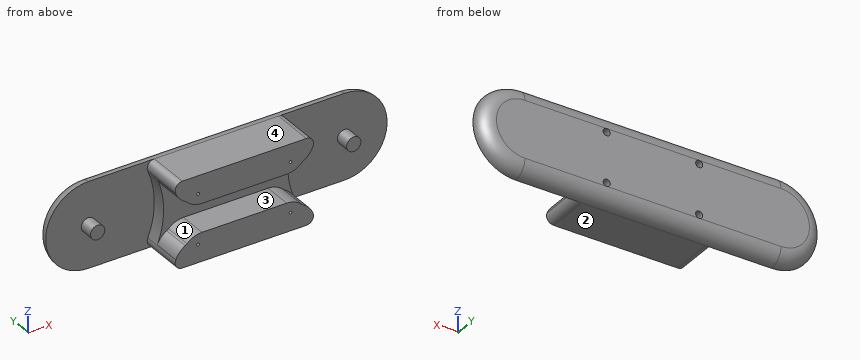
from build123d import *

# Parameters (mm, degrees)
BOSS_EXTRUDE1_DEPTH     = 40
FILLET1_R               = 10
CUT_EXTRUDE1_DEPTH      = 30
SKETCH4_R               = 5
BOSS_EXTRUDE3_DEPTH     = 10
CUT_EXTRUDE2_REACH      = 181.038
CUT_EXTRUDE2_END_RADIUS = 60
SKETCH5_W               = 20
SKETCH5_H               = 40
FILLET2_R               = 5
CUT_EXTRUDE3_REACH      = 153.142
SKETCH6_R               = 1
SKETCH7_R               = 2.5
CUT_EXTRUDE4_DEPTH      = 5
SKETCH8_R               = 6
CUT_EXTRUDE5_DEPTH      = 20
FILLET3_R               = 15


with BuildPart() as part:
    # Sketch1 → Boss-Extrude1 (new body)
    with BuildSketch(Plane(origin=(0, 0, 0), x_dir=(1, 0, 0), z_dir=(0, 1, 0))):
        with BuildLine():
            Line((-67.694698117, 31.515169882), (112.305301883, 31.515169882))
            ThreePointArc((112.305301883, 31.515169882), (142.305301883, 1.515169882), (112.305301883, -28.484830118))
            Line((112.305301883, -28.484830118), (-67.694698117, -28.484830118))
            ThreePointArc((-67.694698117, -28.484830118), (-97.694698117, 1.515169882), (-67.694698117, 31.515169882))
        make_face()
    extrude(amount=BOSS_EXTRUDE1_DEPTH)

    # Fillet1
    fillet1_edges = [part.edges().sort_by_distance(p)[0] for p in [
        (142.305301883, 40, -1.515169882),
        (22.305301883, 40, -31.515169882),
        (-97.694698117, 40, -1.515169882),
        (22.305301883, 40, 28.484830118),
    ]]
    fillet(fillet1_edges, radius=FILLET1_R)

    # Sketch3 → Cut-Extrude1 (cut)
    with BuildSketch(Plane.XZ):
        with BuildLine():
            Line((73.949041486, -31.515169882), (148.949041486, -31.515169882))
            Line((148.949041486, -31.515169882), (148.949041486, 28.484830118))
            Line((148.949041486, 28.484830118), (73.949041486, 28.484830118))
            ThreePointArc((73.949041486, 28.484830118), (65.910565713, -1.515169882), (73.949041486, -31.515169882))
        make_face()
        with BuildLine():
            Line((-29.33843772, 28.484830118), (-104.33843772, 28.484830118))
            Line((-104.33843772, 28.484830118), (-104.33843772, -31.515169882))
            Line((-104.33843772, -31.515169882), (-29.33843772, -31.515169882))
            ThreePointArc((-29.33843772, -31.515169882), (-21.299961947, -1.515169882), (-29.33843772, 28.484830118))
        make_face()
    extrude(amount=-CUT_EXTRUDE1_DEPTH, mode=Mode.SUBTRACT)

    # Sketch4 → Boss-Extrude3 (add)
    with BuildSketch(Plane(origin=(0, 30, 0), x_dir=(-1, 0, 0), z_dir=(0, -1, 0))):
        with Locations(Location((-112.305301883, 1.515169882, 0), (0, 0, 90))):
            Circle(SKETCH4_R)
        with Locations(Location((67.694698117, 1.515169882, 0), (0, 0, 270))):
            Circle(SKETCH4_R)
    extrude(amount=BOSS_EXTRUDE3_DEPTH)

    # Cut-Extrude2: up to this cylinder (the profile starts outside it)
    cut_extrude2_end = Plane(origin=(-81.299961947, 0, -1.515169882), z_dir=(0, -1, 0)) * Cylinder(CUT_EXTRUDE2_END_RADIUS, 483.076, mode=Mode.PRIVATE)
    # Sketch5 → Cut-Extrude2 (cut, up to the surface)
    with BuildSketch(Plane(origin=(73.949041486, 0, 0), x_dir=(0, 0, -1), z_dir=(1, 0, 0)), mode=Mode.PRIVATE) as cut_extrude2_sk1:
        with Locations((1.515169882, 0)):
            Rectangle(SKETCH5_W, SKETCH5_H)
    cut_extrude2_tool1 = extrude(cut_extrude2_sk1.sketch, amount=-CUT_EXTRUDE2_REACH, mode=Mode.PRIVATE) - cut_extrude2_end
    add(cut_extrude2_tool1.solids().sort_by_distance((73.949041, 0, -1.51517))[0], mode=Mode.SUBTRACT)

    # Fillet2
    # the kernel refuses this fillet: 5 mm, written as the material it takes off along each edge
    with BuildSketch(Plane(origin=(-29.33843772, -20.096189432, 28.484830118), x_dir=(0.44322659401027775, 0, -0.8964096085841831), z_dir=(0, 1, 0))) as fillet2_piece_1:
        with BuildLine():
            CenterArc((8.044914281, -4.989633951), FILLET2_R, 93.690067526, 112.619864948)
            Line((3.562866238, -7.205766921), (0, 0))
            ThreePointArc((0, 0), (3.861558855, -0.124392586), (7.72311771, 0))
        make_face()
    extrude(amount=50.096189432, mode=Mode.SUBTRACT)
    with BuildSketch(Plane(origin=(-29.33843772, -20.096189432, -31.515169882), x_dir=(1, 0, 0), z_dir=(0, 1, 0))) as fillet2_piece_2:
        with BuildLine():
            CenterArc((8.038475773, -5), FILLET2_R, 90, 112.619864948)
            ThreePointArc((3.423091158, -6.923076923), (1.823052288, -3.406404359), (0, 0))
            Line((0, 0), (8.038475773, 0))
        make_face()
    extrude(amount=50.096189432, mode=Mode.SUBTRACT)
    with BuildSketch(Plane(origin=(73.949041486, -20.096189432, -31.515169882), x_dir=(-1, 0, 0), z_dir=(0, 1, 0))) as fillet2_piece_3:
        with BuildLine():
            CenterArc((8.038475773, 5), FILLET2_R, 157.380135052, 112.619864948)
            ThreePointArc((3.423091158, 6.923076923), (1.823052288, 3.406404359), (0, 0))
            Line((0, 0), (8.038475773, 0))
        make_face()
    extrude(amount=50.096189432, mode=Mode.SUBTRACT)
    with BuildSketch(Plane(origin=(73.949041486, -20.096189432, 28.484830118), x_dir=(-0.4432265940102763, 0, -0.8964096085841838), z_dir=(0, 1, 0))) as fillet2_piece_4:
        with BuildLine():
            CenterArc((8.044914281, 4.989633951), FILLET2_R, 153.690067526, 112.619864948)
            Line((3.562866238, 7.205766921), (0, 0))
            ThreePointArc((0, 0), (3.861558855, 0.124392586), (7.72311771, 0))
        make_face()
    extrude(amount=50.096189432, mode=Mode.SUBTRACT)

    # Sketch6 → Cut-Extrude3 (cut, up to next)
    with BuildSketch(Plane(origin=(0, 0, 0), x_dir=(-1, 0, 0), z_dir=(0, -1, 0)), mode=Mode.PRIVATE) as cut_extrude3_sk1:
        with Locations(Location((10.194698117, -15.984830118, 0), (0, 0, 90))):
            Circle(SKETCH6_R)
    cut_extrude3_tool1 = extrude(cut_extrude3_sk1.sketch, amount=-CUT_EXTRUDE3_REACH, mode=Mode.PRIVATE) & part.part
    # Sketch6 → Cut-Extrude3 (cut, up to next)
    with BuildSketch(Plane(origin=(0, 0, 0), x_dir=(-1, 0, 0), z_dir=(0, -1, 0)), mode=Mode.PRIVATE) as cut_extrude3_sk2:
        with Locations(Location((-54.805301883, -15.984830118, 0), (0, 0, 90))):
            Circle(SKETCH6_R)
    cut_extrude3_tool2 = extrude(cut_extrude3_sk2.sketch, amount=-CUT_EXTRUDE3_REACH, mode=Mode.PRIVATE) & part.part
    # Sketch6 → Cut-Extrude3 (cut, up to next)
    with BuildSketch(Plane(origin=(0, 0, 0), x_dir=(-1, 0, 0), z_dir=(0, -1, 0)), mode=Mode.PRIVATE) as cut_extrude3_sk3:
        with Locations(Location((-54.805301883, 19.015169882, 0), (0, 0, 90))):
            Circle(SKETCH6_R)
    cut_extrude3_tool3 = extrude(cut_extrude3_sk3.sketch, amount=-CUT_EXTRUDE3_REACH, mode=Mode.PRIVATE) & part.part
    # Sketch6 → Cut-Extrude3 (cut, up to next)
    with BuildSketch(Plane(origin=(0, 0, 0), x_dir=(-1, 0, 0), z_dir=(0, -1, 0)), mode=Mode.PRIVATE) as cut_extrude3_sk4:
        with Locations(Location((10.194698117, 19.015169882, 0), (0, 0, 90))):
            Circle(SKETCH6_R)
    cut_extrude3_tool4 = extrude(cut_extrude3_sk4.sketch, amount=-CUT_EXTRUDE3_REACH, mode=Mode.PRIVATE) & part.part
    add(cut_extrude3_tool1.solids().sort_by_distance((-10.194698, 0, 15.98483))[0], mode=Mode.SUBTRACT)
    add(cut_extrude3_tool2.solids().sort_by_distance((54.805302, 0, 15.98483))[0], mode=Mode.SUBTRACT)
    add(cut_extrude3_tool3.solids().sort_by_distance((54.805302, 0, -19.01517))[0], mode=Mode.SUBTRACT)
    add(cut_extrude3_tool4.solids().sort_by_distance((-10.194698, 0, -19.01517))[0], mode=Mode.SUBTRACT)

    # Sketch7 → Cut-Extrude4 (cut)
    with BuildSketch(Plane(origin=(0, 40, 0), x_dir=(1, 0, 0), z_dir=(0, 1, 0))):
        with Locations(Location((-10.194698117, 19.015169882, 0), (0, 0, 270))):
            Circle(SKETCH7_R)
        with Locations(Location((-10.194698117, -15.984830118, 0), (0, 0, 270))):
            Circle(SKETCH7_R)
        with Locations(Location((54.805301883, -15.984830118, 0), (0, 0, 270))):
            Circle(SKETCH7_R)
        with Locations(Location((54.805301883, 19.015169882, 0), (0, 0, 270))):
            Circle(SKETCH7_R)
    extrude(amount=-CUT_EXTRUDE4_DEPTH, mode=Mode.SUBTRACT)

    # Sketch8 → Cut-Extrude5 (cut)
    with BuildSketch(Plane.XZ):
        with Locations((-22.139164116, 8.484830118)):
            Circle(SKETCH8_R)
        with Locations((-22.139164116, -11.515169882)):
            Circle(SKETCH8_R)
        with Locations((66.749767882, -11.515169882)):
            Circle(SKETCH8_R)
        with Locations((66.749767882, 8.484830118)):
            Circle(SKETCH8_R)
    extrude(amount=-CUT_EXTRUDE5_DEPTH, mode=Mode.SUBTRACT)

    # Fillet3
    fillet3_edges = [part.edges().sort_by_distance(p)[0] for p in [
        (-16.139164116, 10, -11.515169882),
        (60.749767882, 10, -11.515169882),
        (68.044321089, 10, 14.343510174),
        (60.749767882, 10, 8.484830118),
        (68.044321089, 10, -17.373849938),
        (-23.433717323, 10, -17.373849938),
        (-23.433717323, 10, 14.343510174),
        (-16.139164116, 10, 8.484830118),
    ]]
    fillet(fillet3_edges, radius=FILLET3_R)


solid = part.part
Read the model definition and answer for the solid it produces. Units are mm, in the model's axes. Face numbers are marked on the shaded views. Coordinates: 2 decimals unless noted, no trailing zeros. Order: outer loops, then holes, each group sorted by start corner. A loop starts at its lowest first (then second) coordinate and runs counter-clockwise, first axis right, second up. Notation, with made-up numbers: (13.5, 15.25) - (28.5, 15.25) arc R18 ccw to (28.5, 29.25) - close; hole circle Ø1 at (-32, 83). An arc over 180 degrees is marked (long way). Use one line per item in the form item = value.
(1) Section C-C, the plane x = -30.5 is taken. Give the vertices of the cut face in (y, z), then the cut area to 3 significant figures.
Computed values:
outline = (30, -31.52) arc R10 ccw to (40, -21.52) - (40, 18.48) arc R10 ccw to (30, 28.48) - close
area = 557 mm²
(2) Straight lines are drawn through the part: L1, parallel to X at y = 36, z = 16; L2, parallel to X at y = 37.5, z = 15; L3, parallel to Y at x = 69, z = 15. For each, find the intervals that lie inside material, in ascending order.
Computed values:
L1 = -89.54 to -12.69, -7.69 to 52.31, 57.31 to 134.15
L2 = -88.57 to -12.49, -7.9 to 52.51, 57.1 to 133.18
L3 = 30 to 40
(3) Section B-B, the plane y = 27 is taken. Give the vertices of the cut face in (x, z), then the cut area to 3 significant figures.
Computed values:
outline = circle Ø10 at (-67.69, -1.52); (-25.92, -24.59) arc R5 ccw to (-21.3, -31.52) - (65.91, -31.52) arc R5 ccw to (70.53, -24.59) arc R60 cw to (70.53, 21.56) arc R5 ccw to (65.91, 28.48) - (-21.3, 28.48) arc R5 ccw to (-25.92, 21.56) arc R60 cw to start; circle Ø10 at (112.31, -1.52); hole circle Ø2 at (-10.19, -19.02); hole circle Ø2 at (-10.19, 15.98); hole circle Ø2 at (54.81, -19.02); hole circle Ø2 at (54.81, 15.98)
area = 5,630 mm²
(4) Given pin 1 Ø2 at (y, z) = (14, -24.5) entering from -X; pin 2 Ø1 at (x, y) = (35.5, 33.5) entering from +Z; pin 3 Ø4.5 at (x, z) = (54.81, -19.02) entering from +Y, each flat-ended and moving along its own axis, determine where each tip first touches the part or whether it passes through.
Computed values:
pin_1 = -26.2
pin_2 = 28.02
pin_3 = 35
(5) Section A-A, the plane x = 35.5 is taken. Give the vertices of the cut face in (y, z).
Computed values:
outline = (0, -31.52) - (30, -31.52) arc R10 ccw to (40, -21.52) - (40, 18.48) arc R10 ccw to (30, 28.48) - (0, 28.48) - (0, 8.48) - (20, 8.48) - (20, -11.52) - (0, -11.52) - close
(6) For a pull along Z with two mould halves and no side action, classify the marked faces 1, 2, 3 and 4 as pulls with the +Z half, pulls with the -Z half, needs draft (parallel to the pull), parting line crosses it, or undercut.
Computed values:
face_1 = undercut
face_2 = pulls with the -Z half
face_3 = undercut
face_4 = pulls with the +Z half
